```python
from build123d import *

# Parameters (mm, degrees)
SKETCH_1_W          = 40
SKETCH_1_H          = 42
EXTRUDE_1_DEPTH     = 10
SKETCH_2_W          = 44
SKETCH_2_H          = 46
EXTRUDE_2_DEPTH     = 3
FILLET_1_R          = 2
FILLET_2_R          = 2
FILLET_3_R          = 2
FILLET_4_R          = 2
FILLET_5_R          = 2
SKETCH_4_R          = 0.5
CUT_EXTRUDE_1_DEPTH = 3


# Some blends are built 0.0001 mm under size
with BuildPart() as part:
    # 草图1 → 凸台-拉伸1 (new body)
    with BuildSketch(Plane.XY):
        Polygon((-42, -2), (0, -2), (2, -2), (2, 44), (-42, 44), align=None)
        with Locations((-20, 21)):
            Rectangle(SKETCH_1_W, SKETCH_1_H, mode=Mode.SUBTRACT)
    extrude(amount=EXTRUDE_1_DEPTH)

    # 草图2 → 凸台-拉伸2 (add)
    with BuildSketch(Plane.XY):
        with Locations((-20, 21)):
            Rectangle(SKETCH_2_W, SKETCH_2_H)
    extrude(amount=-EXTRUDE_2_DEPTH)

    # 圆角1
    fillet_1_edges = [part.edges().sort_by_distance(p)[0] for p in [
        (-20, 44, -3),
    ]]
    fillet(fillet_1_edges, radius=FILLET_1_R)

    # 圆角2
    fillet_2_edges = [part.edges().sort_by_distance(p)[0] for p in [
        (2, 44, 4.5),
        (2, 20, -3),
        (2, 43.414213562, -2.414213562),
    ]]
    fillet(fillet_2_edges, radius=FILLET_2_R)

    # 圆角3
    fillet_3_edges = [part.edges().sort_by_distance(p)[0] for p in [
        (-42, -2, 3.5),
        (2, -2, 4.5),
        (-21, -2, -3),
        (1.414213562, -2, -2.414213562),
        (-20, -2, 10),
    ]]
    fillet(fillet_3_edges, radius=FILLET_3_R - 0.0001)  # a hair under: the kernel refuses the full size

    # 圆角4
    # the kernel refuses this fillet: 2 mm, written as the material it takes off along each edge
    with BuildSketch(Plane(origin=(0, -2, 8), x_dir=(1, 0, 0), z_dir=(0, 0, -1))) as fillet_4_piece_1:
        with BuildLine():
            CenterArc((0.0001, -1.9999), 1.9999, 0, 90)
            Line((2, -1.9999), (2, 0))
            Line((2, 0), (0.0001, 0))
        make_face()
    revolve(axis=Axis((0, -2, 8), (0, -1, 0)), revolution_arc=90, mode=Mode.SUBTRACT)
    with BuildSketch(Plane(origin=(0, 44, 10), x_dir=(0, -1, 0), z_dir=(-1, 0, 0))) as fillet_4_piece_2:
        with BuildLine():
            CenterArc((FILLET_4_R, -FILLET_4_R), FILLET_4_R, 90, 90)
            Line((0, -FILLET_4_R), (0, 0))
            Line((0, 0), (FILLET_4_R, 0))
        make_face()
    extrude(amount=47, mode=Mode.SUBTRACT)
    with BuildSketch(Plane(origin=(0, 42, 10), x_dir=(0, 1, 0), z_dir=(-1, 0, 0))) as fillet_4_piece_3:
        with BuildLine():
            CenterArc((2 - FILLET_4_R, FILLET_4_R), FILLET_4_R, 270, 90)
            Line((2, FILLET_4_R), (2, 0))
            Line((2, 0), (2 - FILLET_4_R, 0))
        make_face()
    revolve(axis=Axis((0, 42, 10), (0, 0, -1)), revolution_arc=90, mode=Mode.SUBTRACT)
    with BuildSketch(Plane(origin=(2, -2, 10), x_dir=(-1, 0, 0), z_dir=(0, 1, 0))) as fillet_4_piece_4:
        with BuildLine():
            CenterArc((FILLET_4_R, -FILLET_4_R), FILLET_4_R, 90, 90)
            Line((0, -FILLET_4_R), (0, 0))
            Line((0, 0), (FILLET_4_R, 0))
        make_face()
    extrude(amount=44, mode=Mode.SUBTRACT)

    # 圆角5
    # the kernel refuses this fillet: 2 mm, written as the material it takes off along each edge
    with BuildSketch(Plane(origin=(-40, -2, 8), x_dir=(0, 0, 1), z_dir=(1, 0, 0))) as fillet_5_piece_1:
        with BuildLine():
            CenterArc((0.0001, -1.9999), 1.9999, 0, 90)
            Line((2, -1.9999), (2, 0))
            Line((2, 0), (0.0001, 0))
        make_face()
    revolve(axis=Axis((-40, -2, 8), (0, -1, 0)), revolution_arc=90, mode=Mode.SUBTRACT)
    with BuildSketch(Plane(origin=(-40, -2, -1), x_dir=(-1, 0, 0), z_dir=(0, 0, 1))) as fillet_5_piece_2:
        with BuildLine():
            CenterArc((0.0001, -1.9999), 1.9999, 0, 90)
            Line((2, -1.9999), (2, 0))
            Line((2, 0), (0.0001, 0))
        make_face()
    revolve(axis=Axis((-40, -2, -1), (0, -1, 0)), revolution_arc=90, mode=Mode.SUBTRACT)
    with BuildSketch(Plane(origin=(-42, 42, 10), x_dir=(0, 0, -1), z_dir=(0, -1, 0)), Plane(origin=(-42, -2, -3), x_dir=(0, 0, 1), z_dir=(0, 1, 0))) as fillet_5_piece_3:
        with BuildLine():
            CenterArc((FILLET_5_R, FILLET_5_R), FILLET_5_R, 180, 90)
            Line((0, FILLET_5_R), (0, 0))
            Line((0, 0), (FILLET_5_R, 0))
        make_face()
    extrude(amount=44, mode=Mode.SUBTRACT)
    with BuildSketch(Plane(origin=(-42, 42, 8), x_dir=(0, 1, 0), z_dir=(0, 0, -1))) as fillet_5_piece_4:
        with BuildLine():
            CenterArc((2 - FILLET_5_R, FILLET_5_R), FILLET_5_R, 270, 90)
            Line((2, FILLET_5_R), (2, 0))
            Line((2, 0), (2 - FILLET_5_R, 0))
        make_face()
    revolve(axis=Axis((-42, 42, 8), (1, 0, 0)), revolution_arc=90, mode=Mode.SUBTRACT)
    with BuildSketch(Plane(origin=(-42, 44, -1), x_dir=(0, -1, 0), z_dir=(0, 0, 1))) as fillet_5_piece_5:
        with BuildLine():
            CenterArc((FILLET_5_R, FILLET_5_R), FILLET_5_R, 180, 90)
            Line((0, FILLET_5_R), (0, 0))
            Line((0, 0), (FILLET_5_R, 0))
        make_face()
    extrude(amount=9, mode=Mode.SUBTRACT)
    with BuildSketch(Plane(origin=(-42, 42, -1), x_dir=(0, 1, 0), z_dir=(0, 0, 1))) as fillet_5_piece_6:
        with BuildLine():
            CenterArc((2 - FILLET_5_R, -FILLET_5_R), FILLET_5_R, 0, 90)
            Line((2, -FILLET_5_R), (2, 0))
            Line((2, 0), (2 - FILLET_5_R, 0))
        make_face()
    revolve(axis=Axis((-42, 42, -1), (-1, 0, 0)), revolution_arc=90, mode=Mode.SUBTRACT)

    # 草图4 → 切除-拉伸1 (cut)
    with BuildSketch(Plane.XY):
        with Locations((-39, 22)):
            Circle(SKETCH_4_R)
        with Locations((-39, 20)):
            Circle(SKETCH_4_R)
    extrude(amount=-CUT_EXTRUDE_1_DEPTH, mode=Mode.SUBTRACT)


solid = part.part
```
Here's how the part is built. I have some questions about the finished solid (model axes, mm). A direction names the side the tool comes from. Coordinates: 2 decimals unless noted, no trailing zeros. Write each loop counter-clockwise with the first axis right and the second up, starting at its lowest first coordinate (ties: lowest second). Pieces come first, ordered by that corner, then holes. Notation, with made-up numbers: (54, 29) - (81, 29) arc R11 cw to (81, 48) - close; hole circle Ø6 at (73.25, -34). An arc over 180 degrees is marked (long way). One line per item, written item: value.
1) I'm going to push flat-ended pins straight in: P1, Ø1, axis at x = -31, y = 18, coming from the +Z side; P2, Ø2, axis at x = -32, z = 8.5, coming from the +Y side. Where does each tip first touch, or does it pass through?
Model answer:
P1: stops at z = 0
P2: stops at y = 44
2) We'd pull the mould along Y, two halves only. Please class faces 1 (the cylindrical face through (-39.4, 22.3, -1.5)), 2 (the cylindrical face through (-41.4, 43.43, 3.44)), 3 (the flat face through (2, 21, 4)): pulls with the +Y half, pulls with the -Y half, needs draft (parallel to the pull), parting line crosses it, or undercut.
Model answer:
face 1: undercut
face 2: pulls with the +Y half
face 3: needs draft
3) Suppose I cut it at C-C on y = 3. Write out the boundary of the cut face in (x, z), and give its area (3 significant figures).
Model answer:
outline: (-42, -1) arc R2 ccw to (-40, -3) - (0, -3) arc R2 ccw to (2, -1) - (2, 8) arc R2 ccw to (0, 10) - (0, 0) - (-40, 0) - (-40, 10) arc R2 ccw to (-42, 8) - close
area: 169 mm²
4) Suppose I cut it at A-A on z = 2. Write out the boundary of the cut face in (x, y), and give its area (3 significant figures).
Model answer:
outline: (-42, 0) arc R2 ccw to (-40, -2) - (0, -2) arc R2 ccw to (2, 0) - (2, 42) arc R2 ccw to (0, 44) - (-40, 44) arc R2 ccw to (-42, 42) - close; hole (-40, 0) - (0, 0) - (0, 42) - (-40, 42) - close
area: 341 mm²
5) I need wall thicknesses on line 1 along X through (y, z) = (3, 0.25); line 2 along Y through (x, z) = (-39, -1.6); line 3 along Y through (x, z) = (-15, 7). Which ranges of each line are inside material? Lowest first, please.
Model answer:
line 1: x = -42 to -40, 0 to 2
line 2: y = -1.91 to 19.5, 20.5 to 21.5, 22.5 to 43.91
line 3: y = -2 to 0, 42 to 44
6) On a 3-axis mill with a long thin cutter (end or side, diameter ignored), from which of +Z, -Z, +X, -X, +Y, -Y can I reach the whole of each face in a straight line? I mean faces 4 (the cylindrical face through (-41.4, 20.71, -2.43)), 5 (the flat face through (-40, 21, 5)). Say none if no direction works.
Model answer:
face 4: -Z, -X, +Y, -Y
face 5: +Z
